For this review, take the finished solid that the model builds, in its own axes (mm). Face numbers are marked on the shaded views. A direction names the side the tool comes from. Give positions to 0.01 mm unless a question says otherwise; leave off trailing zeros. Order: outer loops, then holes, each group sorted by start corner. A loop starts at its lowest first (then second) coordinate and runs counter-clockwise, first axis right, second up.
Item 1: Machinability: for the marked faces 1 and 2, which of the approach directions +Z, -Z, +X, -X, +Y, -Y give a long, thin tool a straight path to every point of the face, cutting with its end or side? Answer none if there is none.
Item 2: Consider section A-A (x = 0). Give the boundary of the cut face in (y, z) (3 decimals), plus the area to 3 significant figures.
Item 3: Consider section D-D (y = 10). Give the boundary of the cut face in (x, z) (3 decimals).
Item 4: For probe 1 along Z at (x, y) = (0, 8) (3 decimals); probe 2 along Y at (x, z) = (0, -1); probe 3 along X at (y, z) = (24, -4.25), list the stretches that pass through material, from the lowest coordinate up.
Item 5: The part is to be moulded in two halves that separate along X. For the marked faces 3, 4 and 5, say which applies: released by +X, released by -X, zero draft, split by the parting line, or undercut.
Item 6: Consider section B-B (y = 23). Give the boundary of the cut face in (x, z), plus the area to 3 significant figures.
Item 7: For P1, Ø4, axis at x = 3.5, z = 2.5, coming from the -Y side; P2, Ø1.9, axis at x = 0.5, z = 1, coming from the -Y side, all flat-tipped, find the tip position at first contact; note any pin that passes through.
Autodesk Inventor part; units mm, degrees
ref_plane "YZ Plane" through (0, 0, 0) normal (1, 0, 0) x (0, 1, 0)
ref_plane "XZ Plane" through (0, 0, 0) normal (0, 1, 0) x (-1, 0, 0)
ref_plane "XY Plane" through (0, 0, 0) normal (0, 0, 1) x (1, 0, 0)
sketch "Sketch1" plane through (0, 0, 0) normal (0, 1, 0) x (-1, 0, 0)
  circle A0 centre (0, 0) radius 3.175
  line L0 (6.35, 6.35) -> (-6.35, 6.35)
  line L1 (-6.35, 6.35) -> (-6.35, -6.35)
  line L2 (-6.35, -6.35) -> (6.35, -6.35)
  line L3 (6.35, -6.35) -> (6.35, 6.35)
  dimension "d0" = 6.35
  dimension "d1" = 6.35
  dimension "d2" = 6.35
  dimension "d3" = 6.35
extrude "Extrusion1" add sketch "Sketch1" along normal blind 30.1752 contours A0 | L3 L2 L1 L0
extrude "Extrusion2" cut sketch "Sketch1" along normal blind 12.7 contours A0
sketch "Sketch2" plane through (-6.35, 0, 6.35) normal (0, 0, 1) x (1, 0, 0)
  circle A0 centre (6.35, 23.8125) radius 3.3782
  line L0 (12.7, 0) -> (12.7, 30.1752)
  point P0 (6.35, 0)
  dimension "d8" = 6.7564
  dimension "d9" = 23.8125
  dimension "d10" = 6.35
extrude "Extrusion3" cut sketch "Sketch2" against normal blind 12.7
sketch "Sketch3" plane through (0, 30.1752, 0) normal (0, 1, 0) x (1, 0, 0)
  line L0 (6.35, -6.35) -> (6.35, 6.35)
  line L1 (6.35, 6.35) -> (-6.35, 6.35)
  line L2 (-6.35, 6.35) -> (-6.35, -6.35)
  line L3 (-6.35, -6.35) -> (6.35, -6.35)
  point P0 (0, 0)
extrude "Extrusion4" add sketch "Sketch3" along normal blind 3.175
properties part number "clevis"
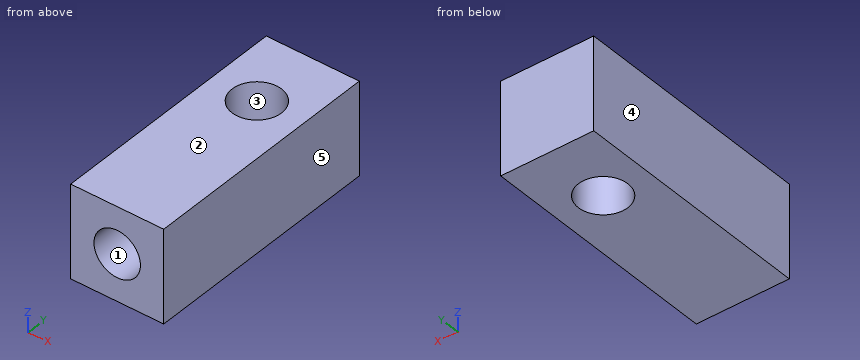
Resolved:
1. face 1: -Y
1. face 2: +Z, +X, -X, +Y, -Y
2. outline: (0, -6.35) - (20.434, -6.35) - (20.434, 6.35) - (0, 6.35) - (0, 3.175) - (12.7, 3.175) - (12.7, -3.175) - (0, -3.175) - close; (27.191, -6.35) - (33.35, -6.35) - (33.35, 6.35) - (27.191, 6.35) - close
2. area: 257 mm2
3. outline: (-6.35, -6.35) - (6.35, -6.35) - (6.35, 6.35) - (-6.35, 6.35) - close; hole circle Ø6.35 at (0, 0)
4. probe 1: z = -6.35 to -3.175, 3.175 to 6.35
4. probe 2: y = 12.7 to 20.43, 27.19 to 33.35
4. probe 3: x = -6.35 to -3.37, 3.37 to 6.35
5. face 3: undercut
5. face 4: released by -X
5. face 5: released by +X
6. outline: (-6.35, -6.35) - (-3.28, -6.35) - (-3.28, 6.35) - (-6.35, 6.35) - close; (3.28, -6.35) - (6.35, -6.35) - (6.35, 6.35) - (3.28, 6.35) - close
6. area: 78.0 mm2
7. P1: stops at y = 0
7. P2: stops at y = 12.7
